```python
from build123d import *

# Parameters (mm, degrees)
SKETCH003_W     = 40
SKETCH003_H     = 100
PAD002_DEPTH    = 20
SKETCH004_W     = 38.4
SKETCH004_H     = 98.4
POCKET001_DEPTH = 19.2
SKETCH006_R     = 5.75
PAD003_DEPTH    = 10
SKETCH009_R     = 5
POCKET004_DEPTH = 10.8
FILLET001_R     = 5
POCKET005_DEPTH = 20.001


with BuildPart() as part:
    # Sketch003 → Pad002 (new body)
    with BuildSketch(Plane.XY):
        Rectangle(SKETCH003_W, SKETCH003_H)
    extrude(amount=PAD002_DEPTH)

    # Sketch004 (on Face6 of Pad002) → Pocket001 (cut)
    with BuildSketch(Plane.XY.offset(20)):
        Rectangle(SKETCH004_W, SKETCH004_H)
    extrude(amount=-POCKET001_DEPTH, mode=Mode.SUBTRACT)

    # Sketch006 (on Face7 of Pocket001) → Pad003 (join)
    with BuildSketch(Plane(origin=(19.2, -2, 0), x_dir=(0, -1, 0), z_dir=(-1, 0, 0))):
        with Locations((25, 6.55)):
            Circle(SKETCH006_R)
    extrude(amount=PAD003_DEPTH)

    # Sketch009 (on Face13 of Pad003) → Pocket004 (cut)
    with BuildSketch(Plane(origin=(9.2, 0, 0), x_dir=(0, -1, 0), z_dir=(-1, 0, 0))):
        with Locations((27, 6.55)):
            Circle(SKETCH009_R)
    extrude(amount=-POCKET004_DEPTH, mode=Mode.SUBTRACT)

    # Fillet001
    fillet001_edges = [part.edges().sort_by_distance(p)[0] for p in [
        (0, 50, 0),
        (0, -50, 0),
        (0, -49.2, 0.8),
        (0, 49.2, 0.8),
    ]]
    fillet(fillet001_edges, radius=FILLET001_R)

    # Sketch010 (on Face4 of Fillet001) → Pocket005 (cut, through all)
    with BuildSketch(Plane.XY.offset(20)):
        Polygon((-20, 50), (-20, -50), (20, -50), (20, -36.2), (0, -36.2), (0, -17.8), (20, -17.8), (20, 50), align=None)
    extrude(amount=-POCKET005_DEPTH, mode=Mode.SUBTRACT)


solid = part.part
```
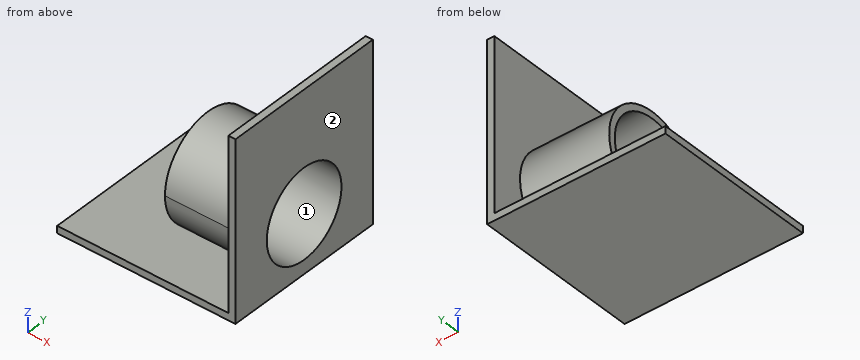
The listing builds one solid part. Answer for the finished solid, in the listing's coordinates (mm). Face numbers are marked on the shaded views. Give positions to 0.01 mm unless a question says otherwise; leave off trailing zeros. Write each loop counter-clockwise with the first axis right and the second up, starting at its lowest first coordinate (ties: lowest second). Pieces come first, ordered by that corner, then holes. Notation, with made-up numbers: (-6, -21.75) -> (8, -21.75) arc R11 cw to (8, -2.75) -> close; hole circle Ø11 at (-20.75, 87). An arc over 180 degrees is marked (long way). Write item = value, one per line. Start each with the question number.
1) Straight lines are drawn through the part: line 1 along Y through (x, z) = (14, 6.75); line 2 along Z through (x, y) = (7.25, -27); line 3 along X through (y, z) = (-29.25, 13.5). For each, find the intervals that lie inside material, in ascending order.
2) The part is cut by section D-D, the plane y = -20.75. Determine the outline of the cut face in (x, z).
3) Determine the mould class of the marked faces 1 and 2 for opening direction Y: +Y half, -Y half, draft (parallel to the pull), parting line (faces both ways), or undercut.
4) The part is cut by section C-C, the plane z = 3. Determine the outline of the cut face in (x, y).
5) The part is cut by section B-B, the plane y = -24.25. Determine the outline of the cut face in (x, z).
6) Each of these flat-tipped pins is pushed along its axis until it touches: pin 1 (9 mm diameter, centred on x = 14, y = -26, fed in from +Z); pin 2 (1 mm diameter, centred on x = 5, z = 3, fed in from -Y); pin 3 (9 mm diameter, centred on y = -26.5, z = 12.5, fed in from -X); pin 4 (5 mm diameter, centred on x = 14, y = -20, fed in from +Z). Where does it stop, or does it pass through?
Solutions:
q1.line_1 = -32.75 to -32, -22 to -21.25
q1.line_2 = 0 to 0.8
q1.line_3 = 19.2 to 20
q2.outline = (0, 0) -> (20, 0) -> (20, 20) -> (19.2, 20) -> (19.2, 0.8) -> (0, 0.8) -> close
q3.face_1 = undercut
q3.face_2 = draft
q4.outline = (9.2, -31.52) -> (19.2, -31.52) -> (19.2, -36.2) -> (20, -36.2) -> (20, -30.52) -> (9.2, -30.52) -> close; (9.2, -23.48) -> (20, -23.48) -> (20, -17.8) -> (19.2, -17.8) -> (19.2, -22.48) -> (9.2, -22.48) -> close
q5.outline = (0, 0) -> (20, 0) -> (20, 2.37) -> (9.2, 2.37) -> (9.2, 1.5) -> (19.2, 1.5) -> (19.2, 0.8) -> (0, 0.8) -> close; (9.2, 10.73) -> (20, 10.73) -> (20, 20) -> (19.2, 20) -> (19.2, 11.6) -> (9.2, 11.6) -> close
q6.pin_1 = 12.3
q6.pin_2 = through
q6.pin_3 = 9.2
q6.pin_4 = 10.13
